```python
from build123d import *

# Parameters (mm, degrees)
F0_W     = 12
F0_H     = 45
F1_DEPTH = 12
F2_W     = 35
F2_H     = 1.2
F3_DEPTH = 12
F4_SIZE  = 5
F5_W     = 8
F5_H     = 31
F6_DEPTH = 1.6
F7_W     = 5
F7_H     = 25
F8_DEPTH = 2.6
F9_R     = 2.49999


# Not quite as in the source:
# - a fillet or chamfer is up to 0.001 mm smaller than in the source, because OpenCascade refuses the exact size


with BuildPart() as f1:
    # F0 (on Top) → F1 (new body)
    with BuildSketch(Plane.XY):
        Rectangle(F0_W, F0_H)
    extrude(amount=F1_DEPTH)

    # F2 (on face) → F3 (cut, through all)
    with BuildSketch(Plane(origin=(-6, 0, 0), x_dir=(0, -1, 0), z_dir=(-1, 0, 0))):
        Polygon((-17.5, 5.4), (17.5, 5.4), (10.9, 12), (-10.9, 12), align=None)
        with Locations((0, 4.8)):
            Rectangle(F2_W, F2_H)
    extrude(amount=-F3_DEPTH, mode=Mode.SUBTRACT)

    # F4
    f4_edges = [f1.edges().sort_by_distance(p)[0] for p in [
        (0, 22.5, 12),
        (0, -22.5, 12),
    ]]
    chamfer(f4_edges, length=F4_SIZE)

    # F5 (on face) → F6 (cut)
    with BuildSketch(Plane.XY.offset(4.2)):
        Rectangle(F5_W, F5_H)
    extrude(amount=-F6_DEPTH, mode=Mode.SUBTRACT)

    # F7 (on face) → F8 (cut, through all)
    with BuildSketch(Plane.XY.offset(2.6)):
        Rectangle(F7_W, F7_H)
    extrude(amount=-F8_DEPTH, mode=Mode.SUBTRACT)

    # F9 (radius 2.5 in the source; OpenCascade refuses exactly that, so slightly less here)
    f9_edges = [f1.edges().sort_by_distance(p)[0] for p in [
        (2.5, 12.5, 1.3),
        (-2.5, 12.5, 1.3),
        (-2.5, -12.5, 1.3),
        (2.5, -12.5, 1.3),
    ]]
    fillet(f9_edges, radius=F9_R)


solid = f1.part
```
Input: part model. Units: mm. Frame: model coordinates. A direction names the side the tool comes from. Give positions to 0.01 mm unless a question says otherwise; leave off trailing zeros. Loops run counter-clockwise (first coordinate to the right, second up) from the corner with the lowest first, then second, coordinate; pieces in that order, holes last. Notation, with made-up numbers: (-8, -30) -> (4, -30) arc R23 ccw to (4, -4) -> close; hole circle Ø2 at (82.5, 48). An arc over 180 degrees is marked (long way). Use a Markdown table: item, result.
Q1. Section query B-B, the plane z = 8. Return the cut outline in (x, y).
Entries:
| item | result |
|---|---|
| outline | (-6, -21.5) -> (6, -21.5) -> (6, -14.9) -> (-6, -14.9) -> close; (-6, 14.9) -> (6, 14.9) -> (6, 21.5) -> (-6, 21.5) -> close |
Q2. Section query A-A, the plane x = -2. Return the cut outline in (y, z).
Entries:
| item | result |
|---|---|
| outline | (-22.5, 0) -> (-11.5, 0) -> (-11.5, 2.6) -> (-15.5, 2.6) -> (-15.5, 4.2) -> (-17.5, 4.2) -> (-17.5, 5.4) -> (-10.9, 12) -> (-17.5, 12) -> (-22.5, 7) -> close; (10.9, 12) -> (17.5, 5.4) -> (17.5, 4.2) -> (15.5, 4.2) -> (15.5, 2.6) -> (11.5, 2.6) -> (11.5, 0) -> (22.5, 0) -> (22.5, 7) -> (17.5, 12) -> close |
Q3. Access query for faces 4 (the flat face through (0, -15.5, 3)), 5 (the flat face through (0, 17.5, 5)), 6 (the flat face through (2.5, 0, 1)). Directions: +Z, -Z, +X, -X, +Y, -Y. A direction counts if a zero-diameter tool reaches every point of the face in a straight line with its end or side. Return the directions, or none.
Entries:
| item | result |
|---|---|
| face 4 | none |
| face 5 | +X, -X |
| face 6 | +Z, -Z |
Q4. Pull-direction query (Y, two-part tool) for faces 1 (the cylindrical face through (1.787, 11.748, 1.282)), 2 (the flat face through (-6, 0, 3)), 3 (the flat face through (-0.1, -20, 9.5)); classes: pulls with the +Y half, pulls with the -Y half, needs draft (parallel to the pull), parting line crosses it, or undercut.
Entries:
| item | result |
|---|---|
| face 1 | undercut |
| face 2 | needs draft |
| face 3 | pulls with the -Y half |
Q5. First-contact query: P1, Ø3.5, axis at x = 0.5, y = 3, coming from the +Z side; P2, Ø2, axis at x = 3.5, z = 9, coming from the +Y side; P3, Ø6.5, axis at x = -2, y = 0.5, coming from the +Z side. Flat tips, straight axial feed; report the tip coordinate or a pass-through.
Entries:
| item | result |
|---|---|
| P1 | passes through |
| P2 | stops at y = 21.5 |
| P3 | stops at z = 4.2 |
Q6. Ray query, probe 1 along Y at (x, z) = (3, 4.5); probe 2 along X at (y, z) = (3, 3.5); probe 3 along X at (y, z) = (-5, 1). Return the intervals inside material, ascending. Write a range as from..to.
Entries:
| item | result |
|---|---|
| probe 1 | y = -22.5..-17.5, 17.5..22.5 |
| probe 2 | x = -6..-4, 4..6 |
| probe 3 | x = -6..-2.5, 2.5..6 |
Q7. Section query C-C, the plane y = 14.5. Return the cut outline in (x, z), plus the area to 3 significant figures.
Entries:
| item | result |
|---|---|
| outline | (-6, 0) -> (6, 0) -> (6, 4.2) -> (4, 4.2) -> (4, 2.6) -> (-4, 2.6) -> (-4, 4.2) -> (-6, 4.2) -> close; (-6, 8.4) -> (6, 8.4) -> (6, 12) -> (-6, 12) -> close |
| area | 80.8 mm² |
Q8. Section query D-D, the plane x = 3.5. Return the cut outline in (y, z).
Entries:
| item | result |
|---|---|
| outline | (-22.5, 0) -> (22.5, 0) -> (22.5, 7) -> (17.5, 12) -> (10.9, 12) -> (17.5, 5.4) -> (17.5, 4.2) -> (15.5, 4.2) -> (15.5, 2.6) -> (-15.5, 2.6) -> (-15.5, 4.2) -> (-17.5, 4.2) -> (-17.5, 5.4) -> (-10.9, 12) -> (-17.5, 12) -> (-22.5, 7) -> close |
